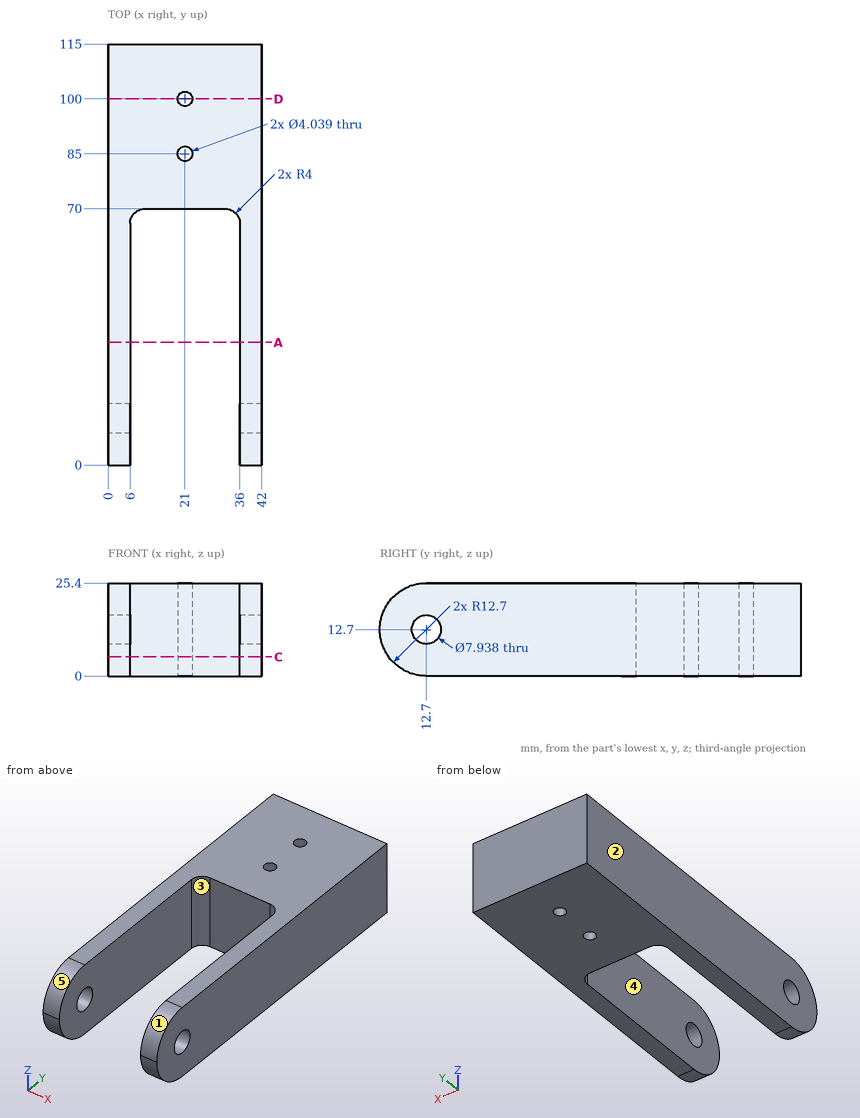
Design review of the part shown in the three views and the two pictorial views. Dimensions are in mm from the part's minimum x, y and z. A direction names the side the tool comes from. Give positions to 0.01 mm unless a question says otherwise; leave off trailing zeros. Order: outer loops, then holes, each group sorted by start corner. A loop starts at its lowest first (then second) coordinate and runs counter-clockwise, first axis right, second up. Notation, with made-up numbers: (-15.5, 87) -> (0.5, 87) arc R19 cw to (0.5, 113) -> close; hole circle Ø9 at (59.5, 29). An arc over 180 degrees is marked (long way). Write each question's results on one line, items separated by ' | '. Start each with the question number.
Q1. Add section A-A on y = 33.5. Give the boundary of the cut face in (x, z), and give its area (3 significant figures).
Q2. For pin 1 (6.5 mm diameter, centred on x = 17, z = 15, fed in from -Y); pin 2 (12 mm diameter, centred on x = 5, z = 19.5, fed in from -Y) (1 decimal), all flat-tipped, find the tip position at first contact; note any pin that passes through.
Q3. Add section C-C on z = 5.25. Give the boundary of the cut face in (x, y) (1 decimal).
Q4. Mouldability with a two-part tool opening along X and no side actions: class the marked faces 1, 2 and 3 as +X half, -X half, draft (parallel to the pull), parting line (faces both ways), or undercut.
Q5. Add section D-D on y = 100. Give the boundary of the cut face in (x, z).
Q6. Machinability: for the marked faces 4 and 5, which of the approach directions +Z, -Z, +X, -X, +Y, -Y give a long, thin tool a straight path to every point of the face, cutting with its end or side? Answer none if there is none.
Q7. Wall thickness on L1, parallel to Y at x = 21, z = 6.5; L2, parallel to X at y = 8.5, z = 1.75; L3, parallel to Y at x = 38.65, z = 12.7: over which ranges is each line inside the solid? List them lowest first. Write a range as from..to.
Found:
1) outline: (0, 0) -> (6, 0) -> (6, 25.4) -> (0, 25.4) -> close; (36, 0) -> (42, 0) -> (42, 25.4) -> (36, 25.4) -> close | area: 305 mm2
2) pin 1: stops at y = 70 | pin 2: stops at y = 0
3) outline: (0, 2.4) -> (6, 2.4) -> (6, 66) arc R4 cw to (10, 70) -> (32, 70) arc R4 cw to (36, 66) -> (36, 2.4) -> (42, 2.4) -> (42, 115) -> (0, 115) -> close; hole circle Ø4 at (21, 85); hole circle Ø4 at (21, 100)
4) face 1: draft | face 2: -X half | face 3: undercut
5) outline: (0, 0) -> (18.98, 0) -> (18.98, 25.4) -> (0, 25.4) -> close; (23.02, 0) -> (42, 0) -> (42, 25.4) -> (23.02, 25.4) -> close
6) face 4: +Z, -Z, -Y | face 5: +Z, +X, -X, -Y
7) L1: y = 70..82.98, 87.02..97.98, 102.02..115 | L2: x = 0..6, 36..42 | L3: y = 0..8.73, 16.67..115
